from build123d import *

# Parameters (mm, degrees)
F0_R     = 2.1
F1_DEPTH = 450


with BuildPart() as f1:
    # F0 (on Front) → F1 (new body)
    with BuildSketch(Plane.XZ):
        with BuildLine():
            Line((4.50066, 1.8), (4.50066, 3.44))
            Line((4.50066, 3.44), (7.16, 6.09934))
            Line((7.16, 6.09934), (12.84, 6.09934))
            Line((12.84, 6.09934), (15.49934, 3.44))
            Line((15.49934, 3.44), (15.49934, 1.8))
            Line((15.49934, 1.8), (12.795146, 1.8))
            Line((12.795146, 1.8), (14.595146, 0))
            Line((14.595146, 0), (18.2, 0))
            ThreePointArc((18.2, 0), (19.472792, 0.527208), (20, 1.8))
            Line((20, 1.8), (20, 5.404854))
            Line((20, 5.404854), (18.2, 7.204854))
            Line((18.2, 7.204854), (18.2, 4.50066))
            Line((18.2, 4.50066), (16.56, 4.50066))
            Line((16.56, 4.50066), (13.90066, 7.16))
            Line((13.90066, 7.16), (13.90066, 12.84))
            Line((13.90066, 12.84), (16.56, 15.49934))
            Line((16.56, 15.49934), (18.2, 15.49934))
            Line((18.2, 15.49934), (18.2, 12.795146))
            Line((18.2, 12.795146), (20, 14.595146))
            Line((20, 14.595146), (20, 18.2))
            ThreePointArc((20, 18.2), (19.472792, 19.472792), (18.2, 20))
            Line((18.2, 20), (14.595146, 20))
            Line((14.595146, 20), (12.795146, 18.2))
            Line((12.795146, 18.2), (15.49934, 18.2))
            Line((15.49934, 18.2), (15.49934, 16.56))
            Line((15.49934, 16.56), (12.84, 13.90066))
            Line((12.84, 13.90066), (7.16, 13.90066))
            Line((7.16, 13.90066), (4.50066, 16.56))
            Line((4.50066, 16.56), (4.50066, 18.2))
            Line((4.50066, 18.2), (7.204854, 18.2))
            Line((7.204854, 18.2), (5.404854, 20))
            Line((5.404854, 20), (1.8, 20))
            ThreePointArc((1.8, 20), (0.527208, 19.472792), (0, 18.2))
            Line((0, 18.2), (0, 14.595146))
            Line((0, 14.595146), (1.8, 12.795146))
            Line((1.8, 12.795146), (1.8, 15.49934))
            Line((1.8, 15.49934), (3.44, 15.49934))
            Line((3.44, 15.49934), (6.09934, 12.84))
            Line((6.09934, 12.84), (6.09934, 7.16))
            Line((6.09934, 7.16), (3.44, 4.50066))
            Line((3.44, 4.50066), (1.8, 4.50066))
            Line((1.8, 4.50066), (1.8, 7.204854))
            Line((1.8, 7.204854), (0, 5.404854))
            Line((0, 5.404854), (0, 1.8))
            ThreePointArc((0, 1.8), (0.527208, 0.527208), (1.8, 0))
            Line((1.8, 0), (5.404854, 0))
            Line((5.404854, 0), (7.204854, 1.8))
            Line((7.204854, 1.8), (4.50066, 1.8))
        make_face()
        Polygon((2.288858, 3.44), (3.349518, 2.37934), (3.349518, 1.8), (1.8, 1.8), (1.8, 3.44), align=None, mode=Mode.SUBTRACT)
        Polygon((18.2, 3.44), (18.2, 1.8), (16.650482, 1.8), (16.650482, 2.37934), (17.711142, 3.44), align=None, mode=Mode.SUBTRACT)
        with Locations((10, 10)):
            Circle(F0_R, mode=Mode.SUBTRACT)
        Polygon((1.8, 16.56), (1.8, 18.2), (3.349518, 18.2), (3.349518, 17.62066), (2.288858, 16.56), align=None, mode=Mode.SUBTRACT)
        Polygon((17.711142, 16.56), (16.650482, 17.62066), (16.650482, 18.2), (18.2, 18.2), (18.2, 16.56), align=None, mode=Mode.SUBTRACT)
    extrude(amount=-F1_DEPTH)


solid = f1.part
Model file for the job. Use its own axes, mm. Give positions to 0.01 mm unless a question says otherwise; leave off trailing zeros. Use one line per item in the form item = value.
(1) Drop flat-ended pins along their axis: P1, Ø4.5, axis at x = 11, y = 268.5, coming from the +Z side; P2, Ø1.5, axis at x = 5, z = 17.5, coming from the +Y side; P3, Ø4, axis at x = 10.5, z = 16.5, coming from the +Y side; P4, Ø1.7, axis at y = 141.5, z = 10, coming from the +X side. Give the stop position or say it passes through.
Determined:
P1 = 18.65
P2 = 450
P3 = through
P4 = 13.9
(2) Drill centre lines: L1, parallel to Z at x = 10, y = 189.5; L2, parallel to X at y = 245.5, z = 6.5; L3, parallel to X at y = 31, z = 2.75. Where is each one in solid material? Low to high.
Determined:
L1 = 6.1 to 7.9, 12.1 to 13.9
L2 = 1.1 to 1.8, 5.44 to 14.56, 18.2 to 18.9
L3 = 0 to 1.8, 2.98 to 4.5, 15.5 to 17.02, 18.2 to 20
(3) Cut at A-A (y = 297). Count the separate pieces of the cut face and the enclosed holes in it, then the cut area to 3 significant figures.
Determined:
separate_pieces = 1
enclosed_holes = 5
area = 161 mm^2
